Input: part model. Units: mm. Frame: model coordinates. Coordinates: 2 decimals unless noted, no trailing zeros. Order: outer loops, then holes, each group sorted by start corner. A loop starts at its lowest first (then second) coordinate and runs counter-clockwise, first axis right, second up. Notation, with made-up numbers: (11, -32) - (28, -32) arc R10 ccw to (28, -24) - close; hole circle Ø10 at (49, -12). An arc over 180 degrees is marked (long way). Answer as CSV lines item,"result". Start each with the question number.
Item 1: Material intervals for line 1 along X through (y, z) = (1.15, 0); line 2 along Z through (x, y) = (-1, 0.5); line 3 along Z through (x, y) = (6, 4.3), sorted ascending.
Item 2: First-contact query: pin 1 (1.5 mm diameter, centred on x = -32.5, y = 3, fed in from -Z); pin 2 (1.5 mm diameter, centred on y = 4, z = -31.5, fed in from -X). Flat tips, straight axial feed; report the tip coordinate or a pass-through.
Item 3: Section C-C (y = 2.25). Output: boundary loops of the cut face in (x, z).
Item 4: Section B-B (z = 0). Output: boundary loops of the cut face in (x, y).
Item 5: Section A-A (x = 0). Output: boundary loops of the cut face in (y, z).
from build123d import *

# Parameters (mm, degrees)
SKETCH_1_R          = 47.5
SKETCH_1_R_2        = 33
EXTRUDE_1_DEPTH     = 5
SKETCH_2_W          = 10
SKETCH_2_H          = 30
CUT_EXTRUDE_1_DEPTH = 25


with BuildPart() as part:
    # Эскиз1 → Бобышка-Вытянуть1 (new body)
    with BuildSketch(Plane(origin=(0, 0, 0), x_dir=(1, 0, 0), z_dir=(0, 1, 0))):
        with Locations(Location((0, 0, 0), (0, 0, 270))):
            Circle(SKETCH_1_R)
        with Locations(Location((0, 0, 0), (0, 0, 270))):
            Circle(SKETCH_1_R_2, mode=Mode.SUBTRACT)
    extrude(amount=EXTRUDE_1_DEPTH)

    # Эскиз2 → Вырез-Вытянуть1 (cut, symmetric)
    with BuildSketch(Plane(origin=(0, 0, 0), x_dir=(0, 0, -1), z_dir=(1, 0, 0))):
        with Locations((-50, 0)):
            Rectangle(SKETCH_2_W, SKETCH_2_H)
        with Locations((50, 0)):
            Rectangle(SKETCH_2_W, SKETCH_2_H)
    extrude(amount=CUT_EXTRUDE_1_DEPTH, both=True, mode=Mode.SUBTRACT)


solid = part.part
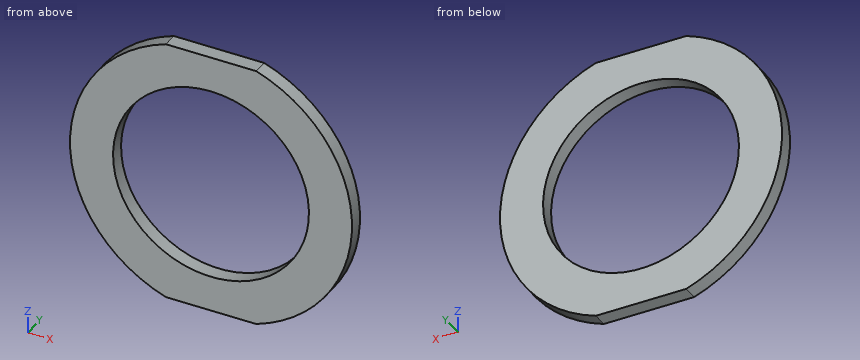
Determined:
1,line 1,"x = -47.5 to -33, 33 to 47.5"
1,line 2,"z = -45 to -32.98, 32.98 to 45"
1,line 3,"z = -45 to -32.45, 32.45 to 45"
2,pin 1,"stops at z = -35.33"
2,pin 2,"stops at x = -36.2"
3,outline,"(-15.21, -45) - (15.21, -45) arc R47.5 ccw to (15.21, 45) - (-15.21, 45) arc R47.5 ccw to start; hole circle Ø66 at (0, 0)"
4,outline,"(-47.5, 0) - (-33, 0) - (-33, 5) - (-47.5, 5) - close; (33, 0) - (47.5, 0) - (47.5, 5) - (33, 5) - close"
5,outline,"(0, -45) - (5, -45) - (5, -33) - (0, -33) - close; (0, 33) - (5, 33) - (5, 45) - (0, 45) - close"
